from build123d import *

# Parameters (mm, degrees)
SKETCH_1_W          = 49
SKETCH_1_H          = 12
SKETCH_1_R          = 3
SKETCH_1_R_2        = 2.5
EXTRUDE_1_DEPTH     = 10
CUT_EXTRUDE_1_DEPTH = 28.133927102
SKETCH_3_R          = 1.5
CUT_EXTRUDE_2_DEPTH = 29.28869032
FILLET_1_R          = 1


with BuildPart() as part:
    # 스케치1 → 보스-돌출1 (new body)
    with BuildSketch(Plane.XY):
        Rectangle(SKETCH_1_W, SKETCH_1_H)
        with Locations((-15, 0)):
            Circle(SKETCH_1_R, mode=Mode.SUBTRACT)
        with Locations(Location((15, 0, 0), (0, 0, 180))):
            Circle(SKETCH_1_R, mode=Mode.SUBTRACT)
        with Locations((-7.5, 0)):
            Circle(SKETCH_1_R_2, mode=Mode.SUBTRACT)
        with Locations(Location((7.5, 0, 0), (0, 0, 180))):
            Circle(SKETCH_1_R_2, mode=Mode.SUBTRACT)
    extrude(amount=EXTRUDE_1_DEPTH)

    # 스케치2 → 컷-돌출1 (cut, through all)
    with BuildSketch(Plane.XY.offset(10)):
        with BuildLine():
            ThreePointArc((-19.330127019, 2.5), (-17.5, 4.330127019), (-15, 5))
            Line((-15, 5), (15, 5))
            ThreePointArc((15, 5), (17.5, 4.330127019), (19.330127019, 2.5))
            Line((19.330127019, 2.5), (24.5, 2.5))
            Line((24.5, 2.5), (24.5, 6))
            Line((24.5, 6), (-24.5, 6))
            Line((-24.5, 6), (-24.5, 2.5))
            Line((-24.5, 2.5), (-19.330127019, 2.5))
        make_face()
        with BuildLine():
            ThreePointArc((-15, -5), (-17.5, -4.330127019), (-19.330127019, -2.5))
            Line((-19.330127019, -2.5), (-24.5, -2.5))
            Line((-24.5, -2.5), (-24.5, -6))
            Line((-24.5, -6), (24.5, -6))
            Line((24.5, -6), (24.5, -2.5))
            Line((24.5, -2.5), (19.330127019, -2.5))
            ThreePointArc((19.330127019, -2.5), (17.5, -4.330127019), (15, -5))
            Line((15, -5), (-15, -5))
        make_face()
        with BuildLine():
            ThreePointArc((-19.898979486, -1), (-20, 0), (-19.898979486, 1))
            Line((-19.898979486, 1), (-24.5, 1))
            Line((-24.5, 1), (-24.5, -1))
            Line((-24.5, -1), (-19.898979486, -1))
        make_face()
        with BuildLine():
            Line((24.5, 1), (19.898979486, 1))
            ThreePointArc((19.898979486, 1), (20, 0), (19.898979486, -1))
            Line((19.898979486, -1), (24.5, -1))
            Line((24.5, -1), (24.5, 1))
        make_face()
        with BuildLine():
            Line((-17.828427125, 1), (-19.898979486, 1))
            ThreePointArc((-19.898979486, 1), (-20, 0), (-19.898979486, -1))
            Line((-19.898979486, -1), (-17.828427125, -1))
            ThreePointArc((-17.828427125, -1), (-18, 0), (-17.828427125, 1))
        make_face()
        with BuildLine():
            ThreePointArc((19.898979486, -1), (20, 0), (19.898979486, 1))
            Line((19.898979486, 1), (17.828427125, 1))
            ThreePointArc((17.828427125, 1), (17.956795679, 0.507305936), (18, 0))
            ThreePointArc((18, 0), (17.956795679, -0.507305936), (17.828427125, -1))
            Line((17.828427125, -1), (19.898979486, -1))
        make_face()
    extrude(amount=-CUT_EXTRUDE_1_DEPTH, mode=Mode.SUBTRACT)

    # 스케치3 → 컷-돌출2 (cut, through all)
    with BuildSketch(Plane(origin=(0, 5, 0), x_dir=(1, 0, 0), z_dir=(0, 1, 0))):
        with Locations((-21.915063509, -2.5)):
            Circle(SKETCH_3_R)
        with Locations((-21.915063509, -7.5)):
            Circle(SKETCH_3_R)
        with Locations(Location((21.915063509, -7.5, 0), (0, 0, 270))):
            Circle(SKETCH_3_R)
        with Locations(Location((21.915063509, -2.5, 0), (0, 0, 270))):
            Circle(SKETCH_3_R)
    extrude(amount=-CUT_EXTRUDE_2_DEPTH, mode=Mode.SUBTRACT)

    # 필렛1
    fillet_1_edges = [part.edges().sort_by_distance(p)[0] for p in [
        (-24.5, 1.75, 10),
        (17.5, 4.330127019, 10),
        (-17.5, 4.330127019, 10),
        (21.915063509, 2.5, 10),
        (-21.915063509, 2.5, 10),
        (0, 5, 10),
        (24.5, -1.75, 10),
        (17.5, -4.330127019, 10),
        (-21.915063509, -2.5, 10),
        (-17.5, -4.330127019, 10),
        (0, -5, 10),
        (21.915063509, -2.5, 10),
        (-24.5, -1.75, 10),
        (24.5, 1.75, 10),
    ]]
    fillet(fillet_1_edges, radius=FILLET_1_R - 0.0001)  # a hair under: the kernel refuses the full size


solid = part.part
Geometry check sheet. Reference: the model listing, model coordinates, mm. A direction names the side the tool comes from. Give positions to 0.01 mm unless a question says otherwise; leave off trailing zeros. Write each loop counter-clockwise with the first axis right and the second up, starting at its lowest first coordinate (ties: lowest second). Pieces come first, ordered by that corner, then holes.
1) Cross-section at B-B (y = 0). Record the boundary of the cut face in (x, z), plus the area to 3 significant figures.
Values follow:
outline: (-12, 0) - (-10, 0) - (-10, 10) - (-12, 10) - close; (-5, 0) - (5, 0) - (5, 10) - (-5, 10) - close; (10, 0) - (12, 0) - (12, 10) - (10, 10) - close
area: 140 mm2
2) Cross-section at C-C (z = 7.5). Count the separate pieces of the cut face and the enclosed holes in it, plus the area to 3 significant figures.
Values follow:
separate pieces: 5
enclosed holes: 2
area: 286 mm2
3) Set-up check for faces 4 (the face through (22, -2.5, 5)), 5 (the face through (-21, -1, 5)), 6 (the face through (22, 2.5, 5)), 7 (the face through (-21.645, -2.199, 9.715)), 8 (the face through (-22, -2.5, 5)): record each of +Z, -Z, +X, -X, +Y, -Y from which the full face is reachable in a straight line by a thin tool's end or side.
Values follow:
face 4: +Z, -Z, +X, -Y
face 5: +Z, -Z, -X
face 6: +Z, -Z, +X, +Y
face 7: +Z, -X, -Y
face 8: +Z, -Z, -X, -Y
4) Release check for a two-part mould opening along Z. For faces 1 (the face through (-21, 1, 5)), 2 (the face through (21.564, -2.199, 9.715)), 3 (the face through (23.18, -1.739, 3.306)) record: released by +Z, released by -Z, zero draft, split by the parting line, or undercut.
Values follow:
face 1: zero draft
face 2: released by +Z
face 3: undercut
5) Thickness scan on line 1 (Y direction, x = 18, z = 2.25); line 2 (Y direction, x = 7.5, z = 8.25); line 3 (X direction, y = 2.75, z = 2.5). Record the ranges inside material, lowest first.
Values follow:
line 1: y = -4 to -1, 1 to 4
line 2: y = -5 to -2.5, 2.5 to 5
line 3: x = -19.18 to -16.2, -13.8 to 13.8, 16.2 to 19.18
6) Go/stop test with flat-tipped pins: pin 1 Ø2.5 at (x, z) = (-22.5, 3.5) entering from -Y; pin 2 Ø1.8 at (x, z) = (21.92, 2.5) entering from -Y; pin 3 Ø6 at (x, y) = (-4.5, -2) entering from -Z; pin 4 Ø3.5 at (x, z) = (-19.5, 7) entering from -Y. Record where each tip stops, or that it passes through.
Values follow:
pin 1: stops at y = -2.5
pin 2: passes through
pin 3: stops at z = 0
pin 4: stops at y = -4.18
7) Cross-section at A-A (z = 5). Record the boundary of the cut face in (x, y).
Values follow:
outline: (-24.5, -2.5) - (-19.33, -2.5) arc R5 ccw to (-15, -5) - (15, -5) arc R5 ccw to (19.33, -2.5) - (24.5, -2.5) - (24.5, -1) - (17.83, -1) arc R3 cw (long way) to (17.83, 1) - (24.5, 1) - (24.5, 2.5) - (19.33, 2.5) arc R5 ccw to (15, 5) - (-15, 5) arc R5 ccw to (-19.33, 2.5) - (-24.5, 2.5) - (-24.5, 1) - (-17.83, 1) arc R3 cw (long way) to (-17.83, -1) - (-24.5, -1) - close; hole circle Ø5 at (-7.5, 0); hole circle Ø5 at (7.5, 0)
